Check sheet for the drawn part. Datum: minimum x, y, z corner. Units: mm. A direction names the side the tool comes from. Give positions to 0.01 mm unless a question says otherwise; leave off trailing zeros. Order: outer loops, then holes, each group sorted by start corner. A loop starts at its lowest first (then second) coordinate and runs counter-clockwise, first axis right, second up. Notation, with made-up numbers: (17.25, -7) - (23.25, -7) arc R26 cw to (23.25, 31) - close; hole circle Ø5 at (37, -22). An arc over 180 degrees is marked (long way). Answer as a JSON object with one key per item and string values. Group by question number.
(1) Section check C-C (x = 16). Record the boundary of the cut face in (y, z), then the cut area to 3 significant figures.
(2) Thickness scan on line 1 (Y direction, x = 25, z = 6.5); line 2 (Z direction, x = 14, y = 4.5); line 3 (Z direction, x = 8.5, y = 3). Record the ranges inside material, lowest first.
(3) Depth check by flat-ended pin: pin 1 Ø3 at (x, y) = (11, 37) entering from +Z; pin 2 Ø5 at (x, y) = (28, 10) entering from +Z. Enter the tip coordinate at first touch or a pass-through.
(4) Section check D-D (x = 24). Record the boundary of the cut face in (y, z).
(5) Section check A-A (z = 8.5). Record the boundary of the cut face in (x, y), then the cut area to 3 significant figures.
(6) Mould release check, pull along Y, two halves, no side actions. Record for the marked faces 1, 2 and 3: +Y half, -Y half, draft (parallel to the pull), parting line (faces both ways), or undercut.
(7) Access from +Z, -Z, +X, -X, +Y, -Y to the whole of each face (thin tool, end or side, straight path). Record for the marked faces 4 and 5.
(8) Section check B-B (y = 2). Record the boundary of the cut face in (x, z), then the cut area to 3 significant figures.
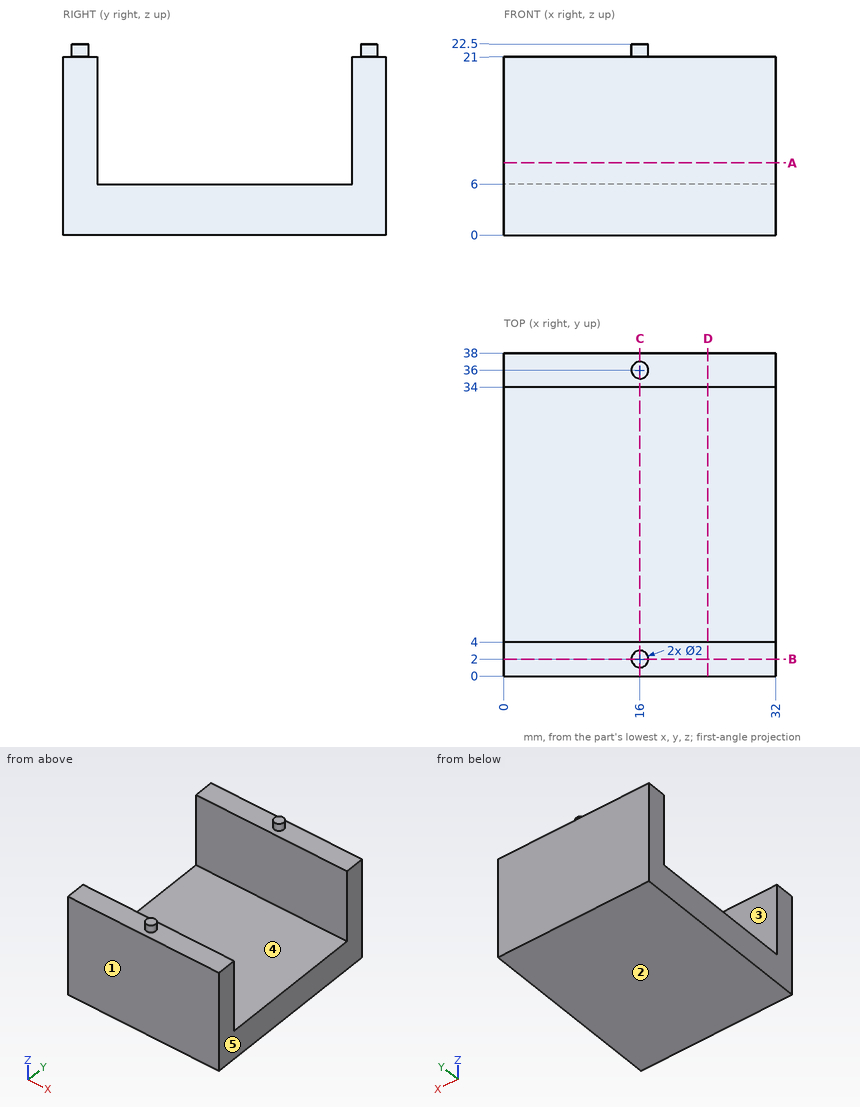
Solutions:
{
 "1": {"outline": "(0, 0) - (38, 0) - (38, 21) - (37, 21) - (37, 22.5) - (35, 22.5) - (35, 21) - (34, 21) - (34, 6) - (4, 6) - (4, 21) - (3, 21) - (3, 22.5) - (1, 22.5) - (1, 21) - (0, 21) - close", "area": "354 mm2"},
 "2": {"line 1": "y = 0 to 4, 34 to 38", "line 2": "z = 0 to 6", "line 3": "z = 0 to 21"},
 "3": {"pin 1": "stops at z = 21", "pin 2": "stops at z = 6"},
 "4": {"outline": "(0, 0) - (38, 0) - (38, 21) - (34, 21) - (34, 6) - (4, 6) - (4, 21) - (0, 21) - close"},
 "5": {"outline": "(0, 0) - (32, 0) - (32, 4) - (0, 4) - close; (0, 34) - (32, 34) - (32, 38) - (0, 38) - close", "area": "256 mm2"},
 "6": {"face 1": "-Y half", "face 2": "draft", "face 3": "undercut"},
 "7": {"face 4": "+Z, +X, -X", "face 5": "+Z, -Z, +X, +Y, -Y"},
 "8": {"outline": "(0, 0) - (32, 0) - (32, 21) - (17, 21) - (17, 22.5) - (15, 22.5) - (15, 21) - (0, 21) - close", "area": "675 mm2"}
}
